```python
from build123d import *

# Parameters (mm, degrees)
SKETCH058_R     = 2.3
PAD040_DEPTH    = 3
PAD041_DEPTH    = 1.5
SKETCH060_R     = 1.25
POCKET011_DEPTH = 0.6
CHAMFER005_SIZE = 0.1


with BuildPart() as part:
    # Sketch058 → Pad040 (new body)
    with BuildSketch(Plane.XY):
        Circle(SKETCH058_R)
    extrude(amount=PAD040_DEPTH)

    # Sketch059 (on Face3 of Pad040) → Pad041 (join)
    with BuildSketch(Plane.XY.offset(3)):
        with BuildLine():
            Line((0.425, 2.767558), (0.425, 3.617558))
            Line((0.425, 3.617558), (-0.425, 3.617558))
            Line((-0.425, 3.617558), (-0.425, 2.767558))
            ThreePointArc((-0.425, 2.767558), (0, -2.8), (0.425, 2.767558))
        make_face()
    extrude(amount=PAD041_DEPTH)

    # Sketch060 → Pocket011 (cut)
    with BuildSketch(Plane.XY):
        Circle(SKETCH060_R)
    extrude(amount=POCKET011_DEPTH, mode=Mode.SUBTRACT)

    # Chamfer005
    chamfer005_edges = [part.edges().sort_by_distance(p)[0] for p in [
        (-1.25, 0, 0),
        (-2.3, 0, 0),
    ]]
    chamfer(chamfer005_edges, length=CHAMFER005_SIZE)


with BuildPart() as part_1:
    # Body017 placement: moved
    add(part.part.moved(Location((63.6, 11.5, -1.5))))


solid = part_1.part
```
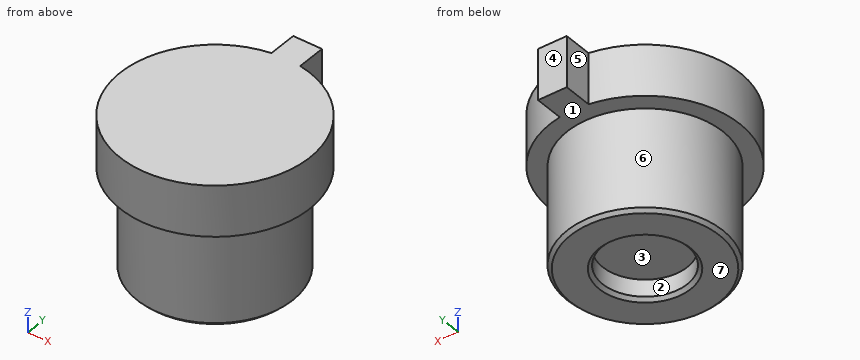
For this review, take the finished solid that the model builds, in its own axes (mm). Face numbers are marked on the shaded views. A direction names the side the tool comes from. Coordinates: 2 decimals unless noted, no trailing zeros. Loops run counter-clockwise (first coordinate to the right, second up) from the corner with the lowest first, then second, coordinate; pieces in that order, holes last. Notation, with made-up numbers: (60.25, 15.5) - (68.25, 15.5) arc R22 ccw to (68.25, 22.5) - close; hole circle Ø6 at (17, -38.75). An arc over 180 degrees is marked (long way). Use one line per item in the form item = value. Start each with the question number.
1) Take a section at D-D (z = 2.3). State the section outline as (x, y) points (3 decimals), plus the area to 3 significant figures.
2) For the marked faces 5, 6 and 7, list the 3-axis set-ups (+Z, -Z, +X, -X, +Y, -Y) from which the entire face can be reached by the end or side of a thin tool; tool diameter is ignored.
3) To check wall thickness, follow probe 1 along Y at (x, z) = (63.6, -1.05); probe 2 along Z at (x, y) = (63.4, 12.25); probe 3 along Z at (x, y) = (61.6, 10.25). State the ranges of each line that lie inside material, in increasing order. Write a range as from..to.
4) Take a section at C-C (z = 1.05). State the section outline as (x, y) points.
5) Take a section at A-A (y = 11.5). State the section outline as (x, z) points, plus the area to 3 significant figures.
6) For pin 1 (0.9 mm diameter, centred on y = 15, z = 2, fed in from +X) (3 decimals); pin 2 (1 mm diameter, centred on x = 63.5, y = 11.5, fed in from -Z); pin 3 (1.5 mm diameter, centred on x = 64.5, z = 0.5, fed in from -Y), all flat-tipped, find the tip position at first contact; note any pin that passes through.
7) Draft analysis for pull direction Y (two halves, no side actions). For the marked faces 1, 2, 3 and 4, state which applies: released by +Y, released by -Y, zero draft, split by the parting line, or undercut.
8) Take a section at B-B (x = 63.6). State the section outline as (y, z) points.
From the geometry:
q1.outline = (63.175, 14.268) arc R2.8 ccw (long way) to (64.025, 14.268) - (64.025, 15.118) - (63.175, 15.118) - close
q1.area = 25.3 mm2
q2.face_5 = +Z, -Z, -X, +Y
q2.face_6 = -Z
q2.face_7 = -Z, +X, -X, +Y, -Y
q3.probe_1 = 9.2..10.25, 12.75..13.8
q3.probe_2 = -0.9..3
q3.probe_3 = 1.5..3
q4.outline = circle Ø4.6 at (63.6, 11.5)
q5.outline = (60.8, 1.5) - (61.3, 1.5) - (61.3, -1.4) - (61.4, -1.5) - (62.25, -1.5) - (62.35, -1.4) - (62.35, -0.9) - (64.85, -0.9) - (64.85, -1.4) - (64.95, -1.5) - (65.8, -1.5) - (65.9, -1.4) - (65.9, 1.5) - (66.4, 1.5) - (66.4, 3) - (60.8, 3) - close
q5.area = 20.7 mm2
q6.pin_1 = 64.025
q6.pin_2 = -0.9
q6.pin_3 = 9.2
q7.face_1 = zero draft
q7.face_2 = undercut
q7.face_3 = undercut
q7.face_4 = released by +Y
q8.outline = (8.7, 1.5) - (9.2, 1.5) - (9.2, -1.4) - (9.3, -1.5) - (10.15, -1.5) - (10.25, -1.4) - (10.25, -0.9) - (12.75, -0.9) - (12.75, -1.4) - (12.85, -1.5) - (13.7, -1.5) - (13.8, -1.4) - (13.8, 1.5) - (15.12, 1.5) - (15.12, 3) - (8.7, 3) - close
